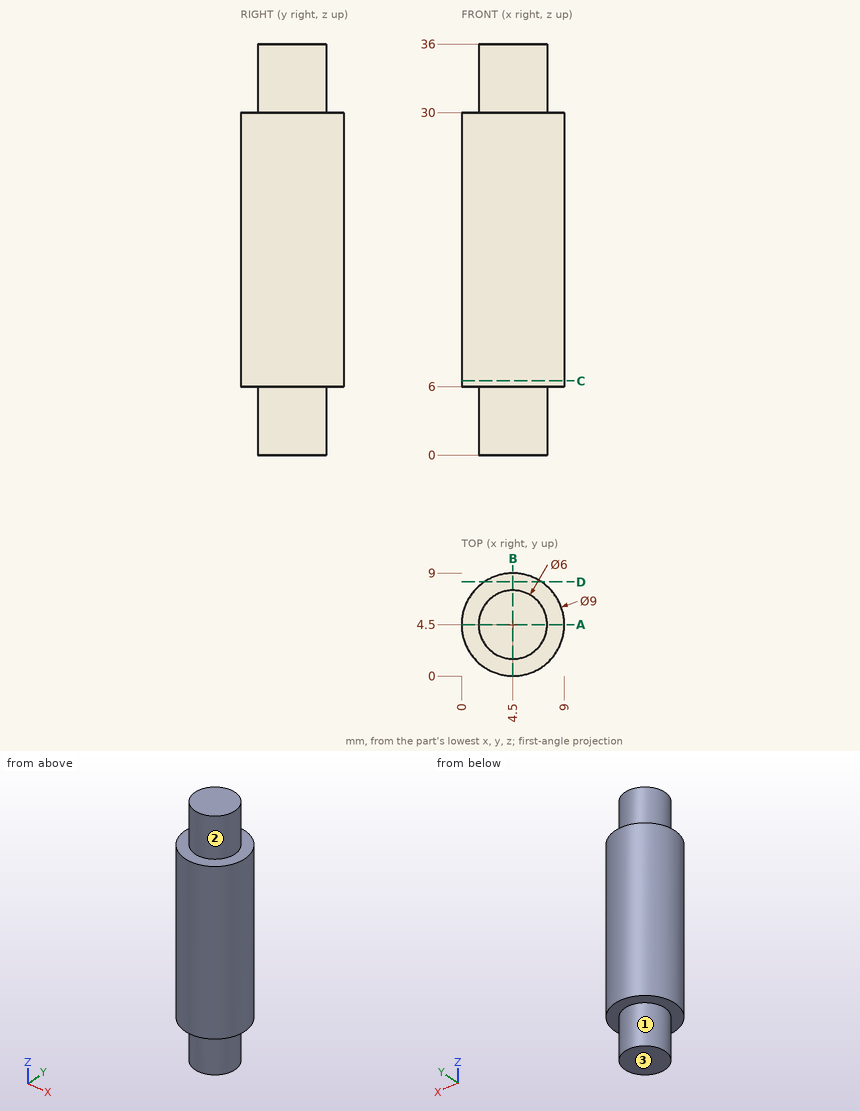
Check sheet for the drawn part. Datum: minimum x, y, z corner. Units: mm. A direction names the side the tool comes from. Coordinates: 2 decimals unless noted, no trailing zeros. Loops run counter-clockwise (first coordinate to the right, second up) from the corner with the lowest first, then second, coordinate; pieces in that order, holes last. Notation, with made-up numbers: (72.5, 35.25) -> (131.5, 35.25) arc R28 cw to (131.5, 65.25) -> close; hole circle Ø7 at (57.25, 34.5). An arc over 180 degrees is marked (long way). Answer as a JSON object with one key per item and string values. Group by question number.
Item 1: Sectioned sample at A-A on y = 4.5. Record the boundary of the cut face in (x, z), plus the area to 3 significant figures.
Item 2: Sectioned sample at C-C on z = 6.5. Record the boundary of the cut face in (x, y).
Item 3: Sectioned sample at D-D on y = 8.25. Record the boundary of the cut face in (x, z), plus the area to 3 significant figures.
Item 4: Scan lines: probe 1 along Z at (x, y) = (7.75, 5.5); probe 2 along X at (y, z) = (7, 34); probe 3 along Y at (x, z) = (5.5, 33.5). Record each from-to range of solid material in increasing order.
Item 5: Depth check by flat-ended pin: pin 1 (3 mm diameter, centred on x = 1.5, z = 8, fed in from +Y); pin 2 (4 mm diameter, centred on y = 7, z = 11.5, fed in from -X); pin 3 (1 mm diameter, centred on x = 2, z = 9, fed in from +Y). Enter the tip coordinate at first touch or a pass-through.
Item 6: Tool access check on the marked faces 1, 2 and 3. Record the directions out of +Z, -Z, +X, -X, +Y, -Y that give a thin tool (end or side, any length) a straight path to the whole face; none if there is none.
Evaluation:
{
 "1": {"outline": "(0, 6) -> (1.5, 6) -> (1.5, 0) -> (7.5, 0) -> (7.5, 6) -> (9, 6) -> (9, 30) -> (7.5, 30) -> (7.5, 36) -> (1.5, 36) -> (1.5, 30) -> (0, 30) -> close", "area": "288 mm²"},
 "2": {"outline": "circle Ø9 at (4.5, 4.5)"},
 "3": {"outline": "(2.01, 6) -> (6.99, 6) -> (6.99, 30) -> (2.01, 30) -> close", "area": "119 mm²"},
 "4": {"probe 1": "z = 6 to 30", "probe 2": "x = 2.84 to 6.16", "probe 3": "y = 1.67 to 7.33"},
 "5": {"pin 1": "stops at y = 8.74", "pin 2": "stops at x = 0.03", "pin 3": "stops at y = 8.53"},
 "6": {"face 1": "-Z", "face 2": "+Z", "face 3": "-Z, +X, -X, +Y, -Y"}
}
